Solid Edge part; units mm, degrees
sketch "Sketch1" plane through (0, 0, 0) normal (0, 0, 1) x (1, 0, 0)
  circle A0 centre (0, 0) radius 80
  circle A1 centre (0, 0) radius 30
  circle A2 centre (70, 0) radius 1.7
  circle A3 centre (49.4975, 49.4975) radius 1.7
  circle A4 centre (0, 70) radius 1.7
  circle A5 centre (-49.4975, 49.4975) radius 1.7
  circle A6 centre (-70, 0) radius 1.7
  circle A7 centre (-49.4975, -49.4975) radius 1.7
  circle A8 centre (0, -70) radius 1.7
  circle A9 centre (49.4975, -49.4975) radius 1.7
  circle A10 centre (40, 0) radius 1.7
  circle A11 centre (20, 34.641) radius 1.7
  circle A12 centre (-20, 34.641) radius 1.7
  circle A13 centre (-40, 0) radius 1.7
  circle A14 centre (-20, -34.641) radius 1.7
  circle A15 centre (20, -34.641) radius 1.7
extrude "Protrusion1" add sketch "Sketch1" along normal blind 6
Could you check a few things on this model? Use its own coordinates, in mm. Round coordinates to 2 decimals unless told otherwise and drop trailing zeros. Write each loop counter-clockwise with the first axis right and the second up, starting at its lowest first coordinate (ties: lowest second). Pieces come first, ordered by that corner, then holes. Notation, with made-up numbers: M -36,58 L -20,58 A21 cw -20,79 Z; hole C 23,18 d11. An arc over 180 degrees is marked long. Answer in a Markdown table with one row per item. Add a question column.
Q1. If we mould it in two halves opening along Y, with no side actions, what happens to faces 1 (the cylindrical face through (-19.086, -36.074, 2.958)), 2 (the cylindrical face through (-17.34, 78.1, 2.96)), 3 (the flat face through (34, 1, 0))? For each: +Y half, -Y half, draft (parallel to the pull), parting line (faces both ways), or undercut.
Q2. Imagine slicing it at B-B (x = -9.5). Please give me the cut outline in (y, z).
Q3. Imagine slicing it at C-C (y = 18). Please give me the cut outline in (x, z), then the cut area to 3 significant figures.
Q4. Imagine slicing it at A-A (z = 2.7). Give the number of separate pieces and of enclosed holes in the cut face, then the cut area to 3 significant figures.
Q5. If I drill on line 1 (Y direction, x = 0, z = 3.45); line 2 (Y direction, x = 20.5, z = 1.5); line 3 (Y direction, x = -35.5, z = 0.6), over which ranges is the centre line in solid material (lowest first)? Write a range as from..to.
Q6. Imagine slicing it at D-D (x = -60). Please give me the cut outline in (y, z), then the cut area to 3 significant figures.
Q7. Will these pins go through, and if not, where does the flat tip stop? pin 1 Ø1 at (x, z) = (-60, 2) entering from +Y; pin 2 Ø2 at (y, z) = (5.5, 4.5) entering from +X.
Values:
| question | item | result |
|---|---|---|
| 1 | face 1 | undercut |
| 1 | face 2 | parting line |
| 1 | face 3 | draft |
| 2 | outline | M -79.43,0 L -28.46,0 L -28.46,6 L -79.43,6 Z; M 28.46,0 L 79.43,0 L 79.43,6 L 28.46,6 Z |
| 3 | outline | M -77.95,0 L -24,0 L -24,6 L -77.95,6 Z; M 24,0 L 77.95,0 L 77.95,6 L 24,6 Z |
| 3 | area | 647 mm^2 |
| 4 | separate pieces | 1 |
| 4 | enclosed holes | 15 |
| 4 | area | 17,200 mm^2 |
| 5 | line 1 | -80..-71.7, -68.3..-30, 30..68.3, 71.7..80 |
| 5 | line 2 | -77.33..-36.27, -33.02..-21.9, 21.9..33.02, 36.27..77.33 |
| 5 | line 3 | -71.69..71.69 |
| 6 | outline | M -52.92,0 L 52.92,0 L 52.92,6 L -52.92,6 Z |
| 6 | area | 635 mm^2 |
| 7 | pin 1 | y = 53.48 |
| 7 | pin 2 | x = 79.87 |
